Geometry: see drawing. Coordinates: mm, zero at the bounding-box minimum. A direction names the side the tool comes from. Give positions to 0.01 mm unless a question says otherwise; leave off trailing zeros. Order: outer loops, then holes, each group sorted by start corner. A loop starts at its lowest first (then second) coordinate and runs counter-clockwise, first axis right, second up. Notation, with made-up numbers: (42, -39) - (59, -39) arc R23 cw to (59, -6) - close; hole circle Ø9 at (-30.75, 77.5). An arc over 180 degrees is marked (long way). Put each result on its own line as item: value. Start each with the question number.
1. Ray query, line 1 along Y through (x, z) = (5, 3.6) (1 decimal); line 2 along Y through (x, z) = (65, 3.85) (1 decimal); line 3 along X through (y, z) = (6, 25). Return the intervals inside material, ascending. Write a range as from..to.
2. Section A-A on z = 45. Return the cut outline in (x, y).
3. Set-up query: the marked faces 5 and 6. Return all of +Z, -Z, +X, -X, +Y, -Y with unobstructed straight access to the full face (end or side cutting, diameter ignored); none if empty.
4. Mould query, pull axis X, two halves, no side actions, for the marked faces 1, 2, 3 and 4. Classes: pulls with the +X half, pulls with the -X half, needs draft (parallel to the pull), parting line crosses it, or undercut.
5. Section C-C on z = 7. Return the cut outline in (x, y).
6. First-contact query: P1, Ø8.5, axis at x = 5, y = 5, coming from the +Z side; P2, Ø1.5, axis at y = 32, z = 49, coming from the -X side; P3, Ø4.5, axis at x = 65, y = 45, coming from the +Z side; P4, Ø2, axis at y = 28, z = 11, coming from the +X side. Flat tips, straight axial feed; report the tip coordinate or a pass-through.
7. Section B-B on y = 85. Return the cut outline in (x, z) (1 decimal).
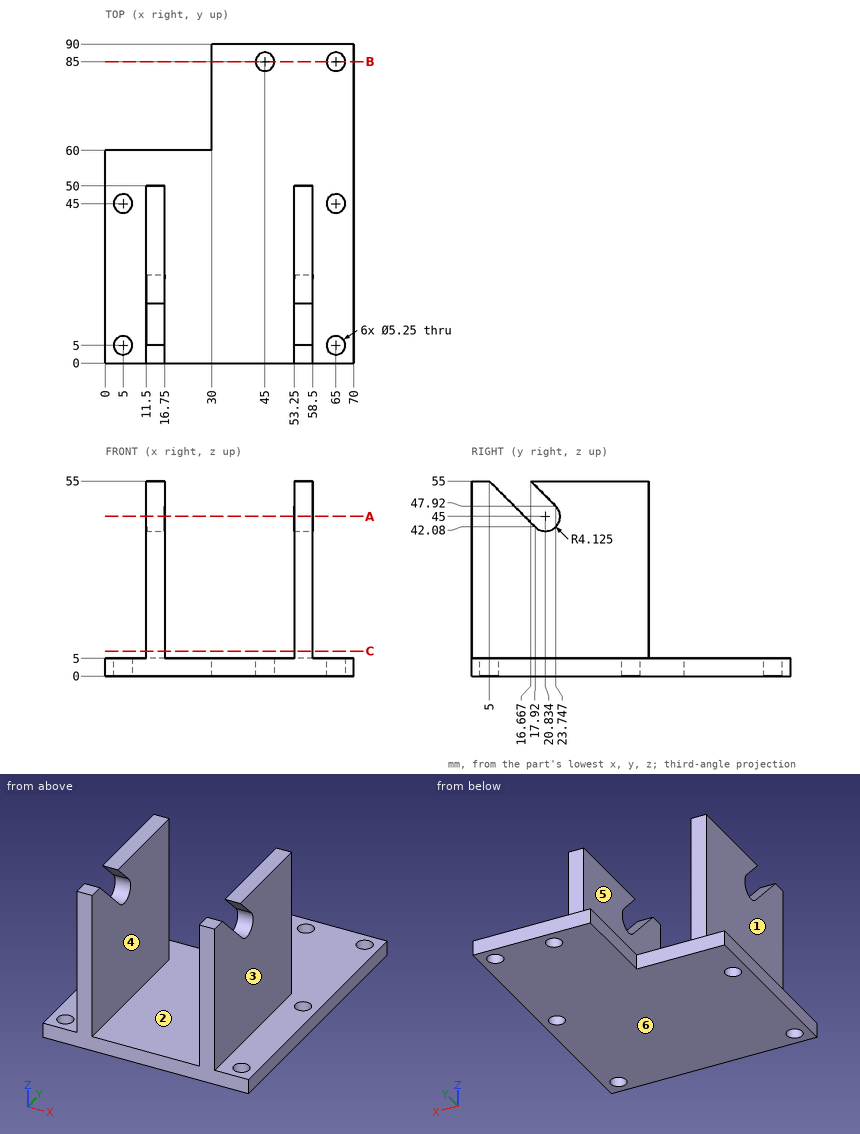
Resolved:
1. line 1: 0..2.4, 7.6..42.4, 47.6..60
1. line 2: 0..2.4, 7.6..42.4, 47.6..82.4, 87.6..90
1. line 3: 11.5..16.75, 53.25..58.5
2. outline: (11.5, 0) - (16.75, 0) - (16.75, 15) - (11.5, 15) - close; (11.5, 24.96) - (16.75, 24.96) - (16.75, 50) - (11.5, 50) - close; (53.25, 0) - (58.5, 0) - (58.5, 15) - (53.25, 15) - close; (53.25, 24.96) - (58.5, 24.96) - (58.5, 50) - (53.25, 50) - close
3. face 5: +Z, +Y, -Y
3. face 6: -Z, +X, -X, +Y, -Y
4. face 1: pulls with the -X half
4. face 2: undercut
4. face 3: pulls with the +X half
4. face 4: undercut
5. outline: (11.5, 0) - (16.75, 0) - (16.75, 50) - (11.5, 50) - close; (53.25, 0) - (58.5, 0) - (58.5, 50) - (53.25, 50) - close
6. P1: z = 5
6. P2: x = 11.5
6. P3: through
6. P4: x = 58.5
7. outline: (30, 0) - (42.4, 0) - (42.4, 5) - (30, 5) - close; (47.6, 0) - (62.4, 0) - (62.4, 5) - (47.6, 5) - close; (67.6, 0) - (70, 0) - (70, 5) - (67.6, 5) - close
